For this review, take the finished solid that the model builds, in its own axes (mm). A direction names the side the tool comes from. Give positions to 0.01 mm unless a question says otherwise; leave off trailing zeros. Order: outer loops, then holes, each group sorted by start corner. A loop starts at its lowest first (then second) coordinate and runs counter-clockwise, first axis right, second up.
Item 1: For P1, Ø1.5, axis at x = 11.5, z = 103.5, coming from the +Y side; P2, Ø4, axis at x = -6, z = 39, coming from the +Y side; P3, Ø12, axis at x = -30.5, y = -5.5, coming from the +Z side; P4, Ø8, axis at x = 3, z = 91, coming from the -Y side, all flat-tipped, find the tip position at first contact; note any pin that passes through.
Item 2: Consider section A-A (z = 89). Give the boundary of the cut face in (x, y), plus the area to 3 significant figures.
Item 3: For probe 1 along X at (y, z) = (-0.5, 50.5); probe 2 along Z at (x, y) = (13.5, 9); probe 3 along Z at (x, y) = (-22, 46), list the stretches that pass through material, from the lowest coordinate up.
Item 4: Machinability: for faces 1 (the cylindrical face through (4.1, -7.89, 63.47)), 2 (the flat face through (1, 1, -5.824)), which of the approach directions +Z, -Z, +X, -X, +Y, -Y give a long, thin tool a straight path to every point of the face, cutting with its end or side? Answer none if there is none.
```python
from build123d import *

# Parameters (mm, degrees)
F0_R     = 8.89
F1_DEPTH = 127
F4_R     = 5.08


with BuildPart() as f1:
    # F0 (on Top) → F1 (new body)
    with BuildSketch(Plane.XY):
        Circle(F0_R)
    extrude(amount=F1_DEPTH)

    # F2 (on Right) → F3 (revolve)
    with BuildSketch(Plane.YZ):
        with BuildLine():
            Line((-50.8, -5.823538), (0, -5.823538))
            Line((0, -5.823538), (0, 0))
            ThreePointArc((0, 0), (-25.811333, 1.355232), (-51.129398, -3.846418))
            ThreePointArc((-51.129398, -3.846418), (-51.802186, -4.974508), (-50.8, -5.823538))
        make_face()
    revolve(axis=Axis((0, 0, -1.317876), (0, 0, 1)))

    # F4
    f4_edges = [f1.edges().sort_by_distance(p)[0] for p in [
        (-8.89, 0, 127),
        (-6.286179, 6.286179, 1.215018),
        (6.286179, -6.286179, 1.215018),
    ]]
    fillet(f4_edges, radius=F4_R)


solid = f1.part
```
Resolved:
1. P1: passes through
1. P2: stops at y = 7.94
1. P3: stops at z = 1.41
1. P4: stops at y = -8.89
2. outline: circle Ø17.78 at (0, 0)
2. area: 248 mm2
3. probe 1: x = -8.88 to 8.88
3. probe 2: z = -5.82 to 1.62
3. probe 3: z = -5.81 to -3.8
4. face 1: +Z
4. face 2: -Z, +X, -X, +Y, -Y
